Can you work these out from the model? Positions are in its coordinate system, mm. A direction names the side the tool comes from. Give positions to 0.01 mm unless a question says otherwise; leave off trailing zeros. Order: outer loops, then holes, each group sorted by start corner. A loop starts at its lowest first (then second) coordinate and runs counter-clockwise, first axis right, second up.
Autodesk Fusion 360 part; units mm, degrees
sketch "Sketch1" plane through (0, 0, 0) normal (0, 0, 1) x (1, 0, 0)
  line L0 (0, 0) -> (44, 0)
  line L1 (44, 0) -> (44, 43.5)
  line L2 (44, 43.5) -> (0, 43.5)
  line L3 (0, 43.5) -> (0, 0)
  dimension "d1" = 44
  dimension "d2" = 43.5
extrude "Extrude1" add sketch "Sketch1" along normal blind 5
sketch "Sketch2" plane through (0, 0, 5) normal (0, 0, 1) x (-1, 0, 0)
  line L0 (0, -43.5) -> (0, 0)
  line L1 (0, 0) -> (-44, 0)
  line L2 (-44, 0) -> (-44, -43.5)
  line L3 (-44, -43.5) -> (0, -43.5)
  line L4 (0, 0) -> (0, -1.25)
  line L5 (0, -1.25) -> (-1.25, -1.25)
  line L6 (-1.25, -1.25) -> (-3.75, -1.25)
  line L7 (-3.75, -1.25) -> (-3.75, -3.541)
  line L8 (-3.75, -3.541) -> (-1.25, -3.541)
  line L9 (-1.25, -3.541) -> (-1.25, -1.25)
  line L10 (-44, 0) -> (-42.75, 0)
  line L11 (-42.75, 0) -> (-42.75, -1.25)
  line L12 (-42.75, -1.25) -> (-40.25, -1.25)
  line L13 (-40.25, -1.25) -> (-40.25, -3.75)
  line L14 (-40.25, -3.75) -> (-42.75, -3.75)
  line L15 (-42.75, -3.75) -> (-42.75, -1.25)
  line L16 (0, -43.5) -> (-1.25, -43.5)
  line L17 (-1.25, -43.5) -> (-1.25, -42.25)
  line L18 (-1.25, -42.25) -> (-3.75, -42.25)
  line L19 (-3.75, -42.25) -> (-3.75, -39.75)
  line L20 (-3.75, -39.75) -> (-1.25, -39.75)
  line L21 (-1.25, -39.75) -> (-1.25, -42.25)
  line L22 (-44, -43.5) -> (-42.75, -43.5)
  line L23 (-42.75, -43.5) -> (-42.75, -42.25)
  line L24 (-42.75, -42.25) -> (-40.25, -42.25)
  line L25 (-40.25, -42.25) -> (-40.25, -39.75)
  line L26 (-40.25, -39.75) -> (-42.75, -39.75)
  line L27 (-42.75, -39.75) -> (-42.75, -42.25)
  dimension "d5" = 1.25
  dimension "d6" = 1.25
  dimension "d7" = 2.5
  dimension "d8" = 1.25
  dimension "d9" = 1.25
  dimension "d10" = 2.5
  dimension "d11" = 2.5
  dimension "d12" = 1.25
  dimension "d13" = 1.25
  dimension "d14" = 2.5
  dimension "d15" = 2.5
  dimension "d16" = 1.25
  dimension "d17" = 1.25
  dimension "d18" = 2.5
  dimension "d19" = 2.5
extrude "Extrude2" cut sketch "Sketch2" against normal blind 1000 contours L6 L7 L8 L9 | L12 L13 L14 L15 | L24 L25 L26 L27 | L18 L19 L20 L21
1) Which directions (+Z, -Z, +X, -X, +Y, -Y) give clear straight access to the entire face, cutting with the end or side of a thin tool? Please do faces 4 (the face through (44, 21, 2)), 5 (the face through (3.75, 2, 3)).
2) We'd pull the mould along X, two halves only. Please class faces 1 (the face through (0, 22, 2)), 2 (the face through (40.25, 2, 3)), 3 (the face through (22, 43.5, 2)): +X half, -X half, draft (parallel to the pull), parting line (faces both ways), or undercut.
3) If I drill on line 1 (Y direction, x = 3.5, z = 3.7); line 2 (X direction, y = 41, z = 4.45), over which ranges is the centre line in solid material (lowest first)?
4) Suppose I cut it at A-A (y = 41.5). Please give me the cut outline in (x, z).
Results:
1. face 4: +Z, -Z, +X, +Y, -Y
1. face 5: +Z, -Z
2. face 1: -X half
2. face 2: undercut
2. face 3: draft
3. line 1: y = 0 to 1.25, 3.54 to 39.75, 42.25 to 43.5
3. line 2: x = 0 to 1.25, 3.75 to 40.25, 42.75 to 44
4. outline: (0, 0) - (1.25, 0) - (1.25, 5) - (0, 5) - close; (3.75, 0) - (40.25, 0) - (40.25, 5) - (3.75, 5) - close; (42.75, 0) - (44, 0) - (44, 5) - (42.75, 5) - close
